from build123d import *

# Parameters (mm, degrees)
F0_W     = 15.875
F0_H     = 15.875
F1_DEPTH = 19.05
F2_R     = 4.7625
F3_DEPTH = 4.826
F4_SIZE  = 1.524
F5_T     = -1.5875


with BuildPart() as f1:
    # F0 (on Front) → F1 (new body)
    with BuildSketch(Plane.XZ):
        Rectangle(F0_W, F0_H)
    extrude(amount=F1_DEPTH)

    # F2 (on face) → F3 (join)
    with BuildSketch(Plane.XZ.offset(19.05)):
        Circle(F2_R)
    extrude(amount=F3_DEPTH)

    # F4
    f4_edges = [f1.edges().sort_by_distance(p)[0] for p in [
        (-4.7625, -23.876, 0),
    ]]
    chamfer(f4_edges, length=F4_SIZE)

    # F5
    f5_openings = [f1.faces().sort_by_distance(p)[0] for p in [
        (0, 0, 0),
    ]]
    offset(amount=F5_T, openings=f5_openings, kind=Kind.INTERSECTION)


solid = f1.part
Input: part model. Units: mm. Frame: model coordinates. A direction names the side the tool comes from. Coordinates: 2 decimals unless noted, no trailing zeros. Loops run counter-clockwise (first coordinate to the right, second up) from the corner with the lowest first, then second, coordinate; pieces in that order, holes last. Notation, with made-up numbers: (4, 43.25) - (56, 43.25) arc R7 cw to (56, 48.25) - close; hole circle Ø9 at (38, 19). An arc over 180 degrees is marked (long way). Answer in a Markdown table with one row per item. Add a question column.
Item 1: Access query for faces 1 (the flat face through (3, -19.05, 4)), 2 (the flat face through (6.35, -9, 0)), 3 (the flat face through (0, -9, 7.938)). Directions: +Z, -Z, +X, -X, +Y, -Y. A direction counts if a zero-diameter tool reaches every point of the face in a straight line with its end or side. Return the directions, or none.
Item 2: Section query A-A on y = -11.75. Return the cut outline in (x, z).
Item 3: Line query: line 1 along Z through (x, y) = (4.5, -14). Output: solid intervals per line, ascending. Write a range as [from, to].
Item 4: Section query B-B on z = 6. Return the cut outline in (x, y), then the cut area to 3 significant figures.
Item 5: Section query C-C on x = 5.5. Return the cut outline in (y, z).
Item 6: Mould query, pull axis Z, two halves, no side actions, for faces 4 (the flat face through (-6.35, -9, 0)), 5 (the flat face through (7.938, -9, 0)), 6 (the flat face through (0, -9, -7.938)), 7 (the cylindrical face through (-3.78, -20.68, -2.9)). Classes: released by +Z, released by -Z, zero draft, split by the parting line, or undercut.
Item 7: Contact query for flat-ended pins moving along their axis: P1, Ø1.5, axis at x = -6, z = -5, coming from the -Y side; P2, Ø2, axis at x = 4.5, z = -2, coming from the +Y side; P3, Ø1.5, axis at x = -1, z = 1, coming from the +Y side. Output: stop coordinate, or through.
Recorded:
| question | item | result |
|---|---|---|
| 1 | face 1 | -Y |
| 1 | face 2 | +Y |
| 1 | face 3 | +Z, +X, -X, +Y, -Y |
| 2 | outline | (-7.94, -7.94) - (7.94, -7.94) - (7.94, 7.94) - (-7.94, 7.94) - close; hole (-6.35, -6.35) - (6.35, -6.35) - (6.35, 6.35) - (-6.35, 6.35) - close |
| 3 | line 1 | [-7.94, -6.35], [6.35, 7.94] |
| 4 | outline | (-7.94, -19.05) - (7.94, -19.05) - (7.94, 0) - (6.35, 0) - (6.35, -17.46) - (-6.35, -17.46) - (-6.35, 0) - (-7.94, 0) - close |
| 4 | area | 80.6 mm^2 |
| 5 | outline | (-19.05, -7.94) - (0, -7.94) - (0, -6.35) - (-17.46, -6.35) - (-17.46, 6.35) - (0, 6.35) - (0, 7.94) - (-19.05, 7.94) - close |
| 6 | face 4 | undercut |
| 6 | face 5 | zero draft |
| 6 | face 6 | released by -Z |
| 6 | face 7 | split by the parting line |
| 7 | P1 | y = -19.05 |
| 7 | P2 | y = -17.46 |
| 7 | P3 | y = -22.29 |
